Model file for the job. Use its own axes, mm. Give positions to 0.01 mm unless a question says otherwise; leave off trailing zeros. Loops run counter-clockwise (first coordinate to the right, second up) from the corner with the lowest first, then second, coordinate; pieces in that order, holes last. Notation, with made-up numbers: M 55.5,39.25 L 114.5,39.25 A36 cw 114.5,74.25 Z; hole C 58.5,37.25 d1. An arc over 180 degrees is marked long. Answer in a Markdown table with one row per item.
```python
from build123d import *

# Parameters (mm, degrees)
EXTRUDE1_DEPTH     = 3.175
CUT_EXTRUDE1_START = -127
SKETCH3_R          = 0.79375
CUT_EXTRUDE1_DEPTH = 203.2


with BuildPart() as part:
    # Sketch1 → Extrude1 (new body)
    with BuildSketch(Plane(origin=(0, 0, 0), x_dir=(1, 0, 0), z_dir=(0, 1, 0))):
        Polygon((25.4, 0), (-25.4, 0), (-25.4, 19.05), (-88.9, 19.05), (-88.9, -10.583333333), (-101.6, -12.7), (-101.6, 25.4), (-19.05, 88.9), (19.05, 88.9), (101.6, 25.4), (101.6, -12.7), (88.9, -10.583333333), (88.9, 19.05), (25.4, 19.05), align=None)
    extrude(amount=EXTRUDE1_DEPTH)

    # Sketch3 → Cut-Extrude1 (cut)
    with BuildSketch(Plane(origin=(25.4, 0, 0), x_dir=(0, 0, -1), z_dir=(1, 0, 0)).offset(CUT_EXTRUDE1_START)):
        with Locations((15.875, 1.5875)):
            Circle(SKETCH3_R)
    extrude(amount=CUT_EXTRUDE1_DEPTH, mode=Mode.SUBTRACT)


solid = part.part
```
Q1. Saw through at A-A (z = -13). Give the cut face in (x, y) (3 decimals), and give its area (3 significant figures).
Reported:
| item | result |
|---|---|
| outline | M -101.6,0 L -88.9,0 L -88.9,3.175 L -101.6,3.175 Z; M -25.4,0 L 25.4,0 L 25.4,3.175 L -25.4,3.175 Z; M 88.9,0 L 101.6,0 L 101.6,3.175 L 88.9,3.175 Z |
| area | 242 mm² |
Q2. Drop flat-ended pins along their axis: pin 1 (1.4 mm diameter, centred on y = 1.59, z = -15.88, fed in from -X); pin 2 (1.6 mm diameter, centred on x = -42, y = 2, fed in from +Z); pin 3 (1 mm diameter, centred on x = 0.5, y = 1.5, fed in from +Z); pin 4 (3 mm diameter, centred on x = -74, z = -32, fed in from -Y). Give the stop position or say it passes through.
Reported:
| item | result |
|---|---|
| pin 1 | through |
| pin 2 | z = -19.05 |
| pin 3 | z = 0 |
| pin 4 | y = 0 |
Q3. Probe probe 1 along X at (y, z) = (2.7, -12.5); probe 2 along X at (y, z) = (2.95, 6); probe 3 along Z at (x, y) = (-4.5, 1.6). List the from-to ranges inside material, lowest first.
Reported:
| item | result |
|---|---|
| probe 1 | -101.6 to -88.9, -25.4 to 25.4, 88.9 to 101.6 |
| probe 2 | -101.6 to -88.9, 88.9 to 101.6 |
| probe 3 | -88.9 to -16.67, -15.08 to 0 |
Q4. Saw through at C-C (x = -85.5). Give the cut face in (y, z) (3 decimals).
Reported:
| item | result |
|---|---|
| outline | M 0,-37.785 L 3.175,-37.785 L 3.175,-19.05 L 0,-19.05 Z |
Q5. Saw through at B-B (z = -34). Give the cut face in (x, y) (3 decimals), and give its area (3 significant figures).
Reported:
| item | result |
|---|---|
| outline | M -90.42,0 L 90.42,0 L 90.42,3.175 L -90.42,3.175 Z |
| area | 574 mm² |
